Design review of the part shown in the three views and the two pictorial views. Dimensions are in mm from the part's minimum x, y and z. A direction names the side the tool comes from. Coordinates: 2 decimals unless noted, no trailing zeros. Loops run counter-clockwise (first coordinate to the right, second up) from the corner with the lowest first, then second, coordinate; pieces in that order, holes last. Notation, with made-up numbers: M 24.5,23 L 80.5,23 A20 ccw 80.5,50 Z; hole C 5,49.5 d8. An arc over 180 degrees is marked long. Use CSV: the item, a comma, the result in double quotes. Start each with the question number.
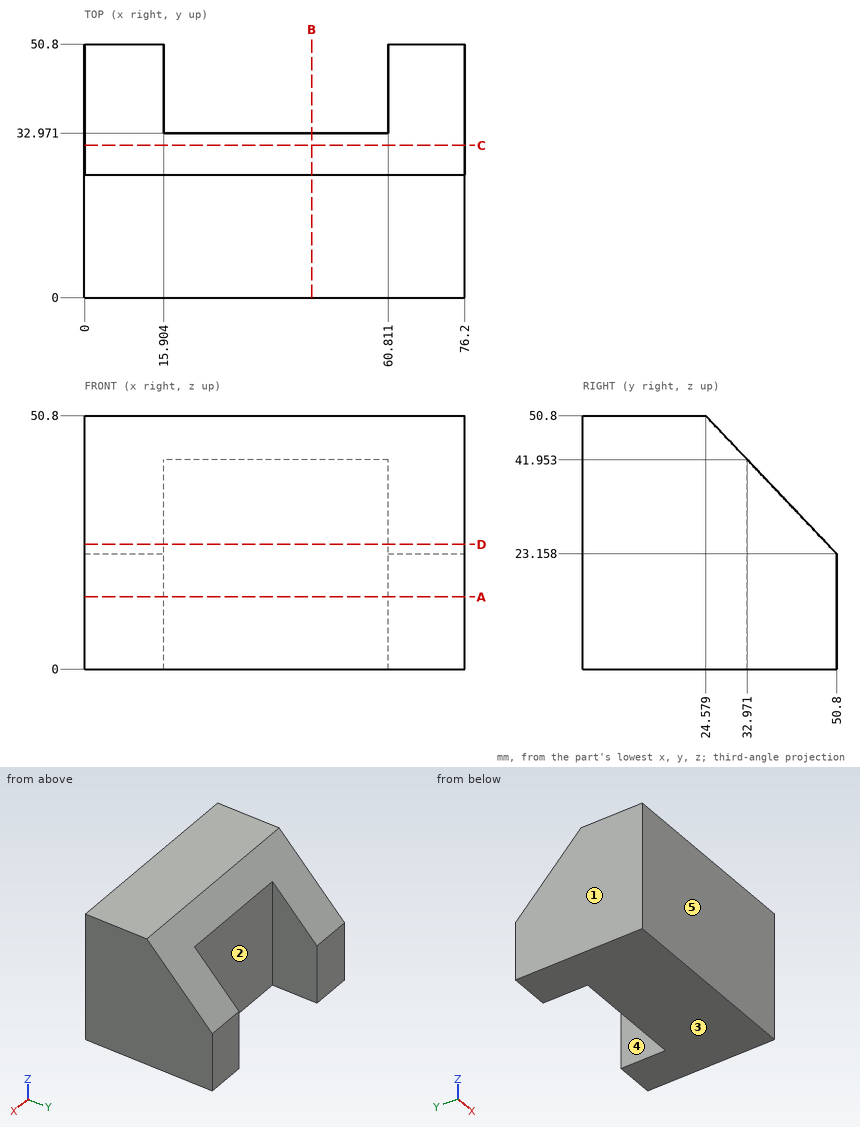
1. For the marked faces 4 and 5, list the 3-axis set-ups (+Z, -Z, +X, -X, +Y, -Y) from which the entire face can be reached by the end or side of a thin tool; tool diameter is ignored.
2. Add section A-A (z = 14.5). Write out the cut boundary in (x, y).
3. Add section B-B (x = 45.5). Write out the cut boundary in (y, z).
4. Insertion check: pin 1 Ø14.5 at (y, z) = (37.5, 23.5) entering from -X; pin 2 Ø3 at (x, z) = (66.5, 25.5) entering from +Y; pin 3 Ø2 at (x, z) = (65.5, 42) entering from +Y (1 decimal); pin 4 Ø1 at (x, z) = (52, 14) entering from +Y. Each pin has a flat end and moves straight along its axis. Give the tip position at first contact, or say it passes through.
5. Add section C-C (y = 30.5). Write out the cut boundary in (x, z).
6. Add section D-D (z = 25). Write out the cut boundary in (x, y), plus the area to 3 significant figures.
7. Draft analysis for pull direction X (two halves, no side actions). For the marked faces 1, 2 and 3, state which applies: released by +X, released by -X, zero draft, split by the parting line, or undercut.
8. To check wall thickness, follow line 1 along X through (y, z) = (39, 34); line 2 along Y through (x, z) = (44, 40); line 3 along Z through (x, y) = (12.5, 44) (1 decimal). State the ranges of each line that lie inside material, in increasing order.
Solved:
1,face 4,"+Z, -Z, +Y"
1,face 5,"+Z, -Z, +X, -X, -Y"
2,outline,"M 0,0 L 76.2,0 L 76.2,50.8 L 60.81,50.8 L 60.81,32.97 L 15.9,32.97 L 15.9,50.8 L 0,50.8 Z"
3,outline,"M 0,0 L 32.97,0 L 32.97,41.95 L 24.58,50.8 L 0,50.8 Z"
4,pin 1,"stops at x = 0"
4,pin 2,"stops at y = 50"
4,pin 3,"stops at y = 33.9"
4,pin 4,"stops at y = 32.97"
5,outline,"M 0,0 L 76.2,0 L 76.2,44.56 L 0,44.56 Z"
6,outline,"M 0,0 L 76.2,0 L 76.2,49.05 L 60.81,49.05 L 60.81,32.97 L 15.9,32.97 L 15.9,49.05 L 0,49.05 Z"
6,area,"3,020 mm^2"
7,face 1,"released by -X"
7,face 2,"undercut"
7,face 3,"zero draft"
8,line 1,"x = 0 to 15.9, 60.81 to 76.2"
8,line 2,"y = 0 to 32.97"
8,line 3,"z = 0 to 30.3"
